Autodesk Inventor part; units mm, degrees
ref_plane "YZ Plane" through (0, 0, 0) normal (1, 0, 0) x (0, 1, 0)
ref_plane "XZ Plane" through (0, 0, 0) normal (0, 1, 0) x (-1, 0, 0)
ref_plane "XY Plane" through (0, 0, 0) normal (0, 0, 1) x (1, 0, 0)
sketch "Boceto1" plane through (0, 0, 0) normal (0, 0, 1) x (1, 0, 0)
  line L0 (-22.5, -22.5) -> (22.5, -22.5)
  line L1 (22.5, -22.5) -> (22.5, 22.5)
  line L2 (22.5, 22.5) -> (-22.5, 22.5)
  line L3 (-22.5, 22.5) -> (-22.5, -22.5)
  line L4 (-22.5, -22.5) -> (22.5, 22.5) construction
  line L5 (22.5, -22.5) -> (-22.5, 22.5) construction
  point P0 (0, 0)
  dimension "d0" = 45
  dimension "d1" = 45
extrude "Extrusión1" add sketch "Boceto1" along normal blind 9
sketch "Boceto2" plane through (0, 0, 9) normal (0, 0, 1) x (1, 0, 0)
  circle A0 centre (0, 0) radius 6
  dimension "d4" = 12
hole "Agujero1" at (0, 0, 9) direction (0, 0, -1) diameter 12 depth 9
sketch "Boceto3" plane through (0, 0, 9) normal (0, 0, 1) x (1, 0, 0)
  line L0 (-15.5, -15.5) -> (15.5, -15.5)
  line L1 (15.5, -15.5) -> (15.5, 15.5)
  line L2 (15.5, 15.5) -> (-15.5, 15.5)
  line L3 (-15.5, 15.5) -> (-15.5, -15.5)
  line L4 (-15.5, -15.5) -> (15.5, 15.5) construction
  line L5 (15.5, -15.5) -> (-15.5, 15.5) construction
  line L6 (0, 15.5) -> (0, -15.5)
  line L7 (-15.5, 0) -> (15.5, 0)
  point P0 (0, 0)
  dimension "d12" = 31
  dimension "d13" = 31
hole "Agujero2" at (-15.5, 15.5, 9) at (-15.5, -15.5, 9) at (15.5, -15.5, 9) at (15.5, 15.5, 9) direction (0, 0, -1) diameter 3 depth 9 tip angle 118
sketch "Boceto4" plane through (0, 0, 0) normal (0, 0, -1) x (-1, 0, 0)
  circle A0 centre (0, 0) radius 12.7
  dimension "d21" = 25.4
extrude "Extrusión2" add sketch "Boceto4" along normal blind 18
properties part number "soporte"
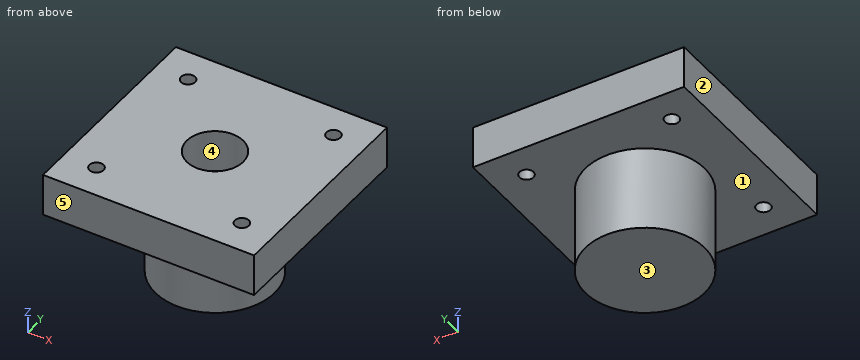
CAD build for the part. Positions are in the model's coordinates, mm. Face numbers are marked on the shaded views. A direction names the side the tool comes from. Coordinates: 2 decimals unless noted, no trailing zeros. Write each loop counter-clockwise with the first axis right and the second up, starting at its lowest first coordinate (ties: lowest second). Pieces come first, ordered by that corner, then holes. Notation, with made-up numbers: (57, 2.5) - (66, 2.5) arc R21 ccw to (66, 32.5) - close; hole circle Ø2 at (74, 13). An arc over 180 degrees is marked (long way). Use a Markdown table: item, result. Add a question column.
Item 1: Mould opens along Y. For the marked faces 3, 4 and 5 say: pulls with the +Y half, pulls with the -Y half, needs draft (parallel to the pull), parting line crosses it, or undercut.
Item 2: Flat gauge pins, fed straight in: pin 1 (1 mm diameter, centred on x = 3, z = -15.5, fed in from +Y); pin 2 (3 mm diameter, centred on y = -10.5, z = -14, fed in from +X); pin 3 (6 mm diameter, centred on x = 1.5, y = 2.5, fed in from +Z); pin 4 (2.5 mm diameter, centred on x = 15.5, y = -15.5, fed in from +Z). Where does each tip first touch, or does it go through?
Item 3: Drill centre lines: L1, parallel to Y at x = -15.5, z = 6; L2, parallel to X at y = 0, z = 2.5. Where is each one in solid material? Low to high. Write a range as from..to.
Item 4: 3-axis set-ups, long thin cutter, end or side, ignore diameter. For the marked faces 1 and 2: which of +Z, -Z, +X, -X, +Y, -Y reach the whole face in a straight line?
Item 5: Band-saw the part on B-B, the plane y = 15.5. Give the cut face in (x, z).
Item 6: Band-saw the part on A-A, the plane z = 3.5. Give the cut face in (x, y).
Item 7: Band-saw the part on D-D, the plane x = 0. Give the cut face in (y, z).
Numbers:
| question | item | result |
|---|---|---|
| 1 | face 3 | needs draft |
| 1 | face 4 | undercut |
| 1 | face 5 | pulls with the -Y half |
| 2 | pin 1 | y = 12.45 |
| 2 | pin 2 | x = 8.96 |
| 2 | pin 3 | z = 0 |
| 2 | pin 4 | through |
| 3 | L1 | -22.5..-17, -14..14, 17..22.5 |
| 3 | L2 | -22.5..-6, 6..22.5 |
| 4 | face 1 | -Z |
| 4 | face 2 | +Z, -Z, -X, +Y, -Y |
| 5 | outline | (-22.5, 0) - (-17, 0) - (-17, 9) - (-22.5, 9) - close; (-14, 0) - (14, 0) - (14, 9) - (-14, 9) - close; (17, 0) - (22.5, 0) - (22.5, 9) - (17, 9) - close |
| 6 | outline | (-22.5, -22.5) - (22.5, -22.5) - (22.5, 22.5) - (-22.5, 22.5) - close; hole circle Ø3 at (-15.5, -15.5); hole circle Ø3 at (-15.5, 15.5); hole circle Ø12 at (0, 0); hole circle Ø3 at (15.5, -15.5); hole circle Ø3 at (15.5, 15.5) |
| 7 | outline | (-22.5, 0) - (-12.7, 0) - (-12.7, -18) - (12.7, -18) - (12.7, 0) - (22.5, 0) - (22.5, 9) - (6, 9) - (6, 0) - (-6, 0) - (-6, 9) - (-22.5, 9) - close |
